```python
from build123d import *

# Parameters (mm, degrees)
CYLINDER127_R             = 10
CYLINDER127_DEPTH         = 170
EXTRUDE010_DEPTH          = 10
FILLET003_R               = 7.72
FILLET003_ROLL_ANGLE      = 90
FILLET003_PLACEMENT_ANGLE = 90
EXTRUDE009_DEPTH          = 10
FILLET002_R               = 7.72
FILLET002_ROLL_ANGLE      = 90
FILLET002_PLACEMENT_ANGLE = 90
CYLINDER237_R             = 2
CYLINDER237_DEPTH         = 42
CYLINDER033_R             = 4
CYLINDER033_DEPTH         = 32
BOX309_W                  = 43
BOX309_H                  = 16
BOX309_DEPTH              = 5
CYLINDER236_R             = 2
CYLINDER236_DEPTH         = 42
CYLINDER034_R             = 4
CYLINDER034_DEPTH         = 32
BOX310_W                  = 43
BOX310_H                  = 16
BOX310_DEPTH              = 5


with BuildPart() as cylinder127:
    # Cylinder127 → Cylinder127 (new body)
    with BuildSketch(Plane(origin=(-119, 28, 146.3), x_dir=(0, 0, -1), z_dir=(1, 0, 0))):
        Circle(CYLINDER127_R)
    extrude(amount=CYLINDER127_DEPTH)


with BuildPart() as fillet003:
    # Wire005 → Extrude010 (new body)
    with BuildSketch(Plane.XY):
        Polygon((0, 0), (16, 0), (56, 150), (40, 150), align=None)
    extrude(amount=EXTRUDE010_DEPTH)

    # Fillet003
    fillet003_edges = [fillet003.edges().sort_by_distance(p)[0] for p in [
        (56, 150, 5),
        (40, 150, 5),
    ]]
    fillet(fillet003_edges, radius=FILLET003_R)


with BuildPart() as fillet003_1:
    # Fillet003 roll: moved
    add(fillet003.part.rotate(Axis((0, 0, 0), (1, 0, 0)), FILLET003_ROLL_ANGLE))


with BuildPart() as fillet003_2:
    # Fillet003 placement: moved
    add(fillet003_1.part.moved(Location((-119, -18, 5))).rotate(Axis((-119, -18, 5), (0, 0, 1)), FILLET003_PLACEMENT_ANGLE))


with BuildPart() as fusion167:
    # Wire004 → Extrude009 (new body)
    with BuildSketch(Plane.XY):
        Polygon((0, 0), (16, 0), (56, 150), (40, 150), align=None)
    extrude(amount=EXTRUDE009_DEPTH)

    # Fillet002
    fillet002_edges = [fusion167.edges().sort_by_distance(p)[0] for p in [
        (56, 150, 5),
        (40, 150, 5),
    ]]
    fillet(fillet002_edges, radius=FILLET002_R)


with BuildPart() as fusion167_1:
    # Fillet002 roll: moved
    add(fusion167.part.rotate(Axis((0, 0, 0), (1, 0, 0)), FILLET002_ROLL_ANGLE))


with BuildPart() as fusion167_2:
    # Fillet002 placement: moved
    add(fusion167_1.part.moved(Location((41, -18, 5))).rotate(Axis((41, -18, 5), (0, 0, 1)), FILLET002_PLACEMENT_ANGLE))

    # Fusion167: union Cylinder127, Fillet003
    add(cylinder127.part)
    add(fillet003_2.part)


with BuildPart() as cylinder237:
    # Cylinder237 → Cylinder237 (new body)
    with BuildSketch(Plane(origin=(17.2, -10, -5), x_dir=(1, 0, 0), z_dir=(0, 0, 1))):
        Circle(CYLINDER237_R)
    extrude(amount=CYLINDER237_DEPTH)


with BuildPart() as cylinder033:
    # Cylinder033 → Cylinder033 (new body)
    with BuildSketch(Plane(origin=(30.2, -10, 0), x_dir=(1, 0, 0), z_dir=(0, 0, 1))):
        Circle(CYLINDER033_R)
    extrude(amount=CYLINDER033_DEPTH)


with BuildPart() as cut203:
    # Box309 → Box309 (new body)
    with BuildSketch(Plane(origin=(8, -18, 0), x_dir=(1, 0, 0), z_dir=(0, 0, 1))):
        with Locations((21.5, 8)):
            Rectangle(BOX309_W, BOX309_H)
    extrude(amount=BOX309_DEPTH)

    # Cut187: cut Cylinder033
    add(cylinder033.part, mode=Mode.SUBTRACT)

    # Cut203: cut Cylinder237
    add(cylinder237.part, mode=Mode.SUBTRACT)


with BuildPart() as cylinder236:
    # Cylinder236 → Cylinder236 (new body)
    with BuildSketch(Plane(origin=(-85, -10, -5), x_dir=(1, 0, 0), z_dir=(0, 0, 1))):
        Circle(CYLINDER236_R)
    extrude(amount=CYLINDER236_DEPTH)


with BuildPart() as cylinder034:
    # Cylinder034 → Cylinder034 (new body)
    with BuildSketch(Plane(origin=(-98, -10, 0), x_dir=(1, 0, 0), z_dir=(0, 0, 1))):
        Circle(CYLINDER034_R)
    extrude(amount=CYLINDER034_DEPTH)


with BuildPart() as fusion169:
    # Box310 → Box310 (new body)
    with BuildSketch(Plane(origin=(-119, -18, 0), x_dir=(1, 0, 0), z_dir=(0, 0, 1))):
        with Locations((21.5, 8)):
            Rectangle(BOX310_W, BOX310_H)
    extrude(amount=BOX310_DEPTH)

    # Cut183: cut Cylinder034
    add(cylinder034.part, mode=Mode.SUBTRACT)

    # Cut202: cut Cylinder236
    add(cylinder236.part, mode=Mode.SUBTRACT)

    # Fusion169: union Fusion167, Cut203
    add(fusion167_2.part)
    add(cut203.part)


with BuildPart() as fusion169_1:
    # Fusion169 placement: moved
    add(fusion169.part.moved(Location((0, 0, 20.1))))


solid = fusion169_1.part
```
Geometry check sheet. Reference: the model listing, model coordinates, mm. A direction names the side the tool comes from. Coordinates: 2 decimals unless noted, no trailing zeros. Loops run counter-clockwise (first coordinate to the right, second up) from the corner with the lowest first, then second, coordinate; pieces in that order, holes last. Notation, with made-up numbers: (51, -19.5) -> (69, -19.5) arc R35 cw to (69, 17.5) -> close; hole circle Ø5 at (6, -30.75). An arc over 180 degrees is marked (long way). Put each result on its own line as item: value.
1) Cross-section at B-B on z = 98. Record the boundary of the cut face in (x, y), plus the area to 3 significant figures.
Result set:
outline: (-119, 1.44) -> (-109, 1.44) -> (-109, 17.44) -> (-119, 17.44) -> close; (41, 1.44) -> (51, 1.44) -> (51, 17.44) -> (41, 17.44) -> close
area: 320 mm^2
2) Tool access check on faces 4 (the flat face through (24, -10, 25.1)), 5 (the cylindrical face through (-35.19, 34.76, 173.77)), 6 (the flat face through (-76, -10, 23)), 7 (the flat face through (-98, -2, 23)). Record the directions out of +Z, -Z, +X, -X, +Y, -Y that give a thin tool (end or side, any length) a straight path to the whole face; none if there is none.
Result set:
face 4: +Z, +Y, -Y
face 5: none
face 6: +Z, -Z, +Y, -Y
face 7: -Z, +X, -X, +Y
3) Thickness scan on line 1 (X direction, y = -10, z = 22); line 2 (X direction, y = 15, z = 102); line 3 (Y direction, x = 30, z = 21) (3 decimals). Record the ranges inside material, lowest first.
Result set:
line 1: x = -119 to -102, -94 to -87, -83 to -76, 8 to 15.2, 19.2 to 26.2, 34.2 to 51
line 2: x = -119 to -109, 41 to 51
line 3: y = -18 to -13.995, -6.005 to -2
4) Cross-section at A-A on x = -85. Record the boundary of the cut face in (y, z).
Result set:
outline: (-18, 20.1) -> (-12, 20.1) -> (-12, 25.1) -> (-18, 25.1) -> close; (-8, 20.1) -> (-2, 20.1) -> (-2, 25.1) -> (-8, 25.1) -> close; circle Ø20 at (28, 166.4)
5) Gauge pin test, flat ends, axial feed: pin 1 Ø5.5 at (x, z) = (-101, 23.5) entering from +Y; pin 2 Ø10.5 at (x, y) = (-98, -10) entering from +Z; pin 3 Ø15.5 at (y, z) = (19, 98) entering from +X; pin 4 Ø3 at (x, y) = (-85, -10) entering from +Z. Record the tip position at first contact, or that the pin passes through.
Result set:
pin 1: stops at y = -2
pin 2: stops at z = 25.1
pin 3: stops at x = 51
pin 4: passes through
6) Release check for a two-part mould opening along X. For faces 1 (the flat face through (51, 4, 98)), 2 (the flat face through (-103, -10, 20.1)), 3 (the cylindrical face through (-102, -10, 23)) record: released by +X, released by -X, zero draft, split by the parting line, or undercut.
Result set:
face 1: released by +X
face 2: zero draft
face 3: undercut
7) Cross-section at C-C on y = -10. Record the boundary of the cut face in (x, z), plus the area to 3 significant figures.
Result set:
outline: (-119, 20.1) -> (-102, 20.1) -> (-102, 25.1) -> (-109, 25.1) -> (-109, 55.1) -> (-119, 55.1) -> close; (-94, 20.1) -> (-87, 20.1) -> (-87, 25.1) -> (-94, 25.1) -> close; (-83, 20.1) -> (-76, 20.1) -> (-76, 25.1) -> (-83, 25.1) -> close; (8, 20.1) -> (15.2, 20.1) -> (15.2, 25.1) -> (8, 25.1) -> close; (19.2, 20.1) -> (26.2, 20.1) -> (26.2, 25.1) -> (19.2, 25.1) -> close; (34.2, 20.1) -> (51, 20.1) -> (51, 55.1) -> (41, 55.1) -> (41, 25.1) -> (34.2, 25.1) -> close
area: 910 mm^2
8) Cross-section at D-D on y = 10.5. Record the boundary of the cut face in (x, z) (3 decimals).
Result set:
outline: (-119, 71.975) -> (-109, 71.975) -> (-109, 131.975) -> (-119, 131.975) -> close; (41, 71.975) -> (51, 71.975) -> (51, 131.975) -> (41, 131.975) -> close
